Read the model definition and answer for the solid it produces. Units are mm, in the model's axes. Face numbers are marked on the shaded views. A direction names the side the tool comes from. Coordinates: 2 decimals unless noted, no trailing zeros. Loops run counter-clockwise (first coordinate to the right, second up) from the corner with the lowest first, then second, coordinate; pieces in that order, holes last. Notation, with made-up numbers: M -28,-35 L 22,-35 A26 ccw 22,-1 Z; hole C 19,52.25 d7. An arc over 180 degrees is marked long. Put each result on its own line as item: value.
from build123d import *

# Parameters (mm, degrees)
BOSS_EXTRUDE1_DEPTH = 46
BOSS_EXTRUDE2_DEPTH = 2
LPATTERN1_COUNT     = 6
LPATTERN1_PITCH     = 7.5
SKETCH3_W           = 10
SKETCH3_H           = 4
BOSS_EXTRUDE3_DEPTH = 8
CUT_EXTRUDE1_REACH  = 6
SKETCH4_R           = 1.55
FILLET1_R           = 3


with BuildPart() as part:
    # Sketch1 → Boss-Extrude1 (new body)
    with BuildSketch(Plane.XY):
        Polygon((0, 0), (0, 42), (-10, 42), (-20, 0), align=None)
    extrude(amount=BOSS_EXTRUDE1_DEPTH)

    # Sketch2 → Boss-Extrude2 (add)
    with BuildSketch(Plane.XY.offset(42.75)):
        with BuildLine():
            Line((-10.595238095, 39.5), (-20.5, 39.5))
            ThreePointArc((-20.5, 39.5), (-21.560660172, 39.060660172), (-22, 38))
            Line((-22, 38), (-22, 1.5))
            ThreePointArc((-22, 1.5), (-21.560660172, 0.439339828), (-20.5, 0))
            Line((-20.5, 0), (-20, 0))
            Line((-20, 0), (-10.595238095, 39.5))
        make_face()
    boss_extrude2 = extrude(amount=-BOSS_EXTRUDE2_DEPTH)

    # LPattern1: Boss-Extrude2 ×6
    with Locations(*[(0, 0, -i * LPATTERN1_PITCH) for i in range(1, LPATTERN1_COUNT)]):
        add(boss_extrude2)

    # Sketch3 → Boss-Extrude3 (add, symmetric)
    with BuildSketch(Plane.XY.offset(23)):
        with Locations((5, 2)):
            Rectangle(SKETCH3_W, SKETCH3_H)
    extrude(amount=BOSS_EXTRUDE3_DEPTH, both=True)

    # Sketch4 → Cut-Extrude1 (cut, up to next)
    with BuildSketch(Plane(origin=(0, 4, 0), x_dir=(1, 0, 0), z_dir=(0, 1, 0)), mode=Mode.PRIVATE) as cut_extrude1_sk1:
        with Locations((5, -19)):
            Circle(SKETCH4_R)
    cut_extrude1_tool1 = extrude(cut_extrude1_sk1.sketch, amount=-CUT_EXTRUDE1_REACH, mode=Mode.PRIVATE) & part.part
    add(cut_extrude1_tool1.solids().sort_by_distance((5, 4, 19))[0], mode=Mode.SUBTRACT)
    # Sketch4 → Cut-Extrude1 (cut, up to next)
    with BuildSketch(Plane(origin=(0, 4, 0), x_dir=(1, 0, 0), z_dir=(0, 1, 0)), mode=Mode.PRIVATE) as cut_extrude1_sk2:
        with Locations((5, -27)):
            Circle(SKETCH4_R)
    cut_extrude1_tool2 = extrude(cut_extrude1_sk2.sketch, amount=-CUT_EXTRUDE1_REACH, mode=Mode.PRIVATE) & part.part
    add(cut_extrude1_tool2.solids().sort_by_distance((5, 4, 27))[0], mode=Mode.SUBTRACT)

    # Fillet1
    fillet1_edges = [part.edges().sort_by_distance(p)[0] for p in [
        (10, 2, 15),
        (10, 2, 31),
    ]]
    fillet(fillet1_edges, radius=FILLET1_R)


solid = part.part
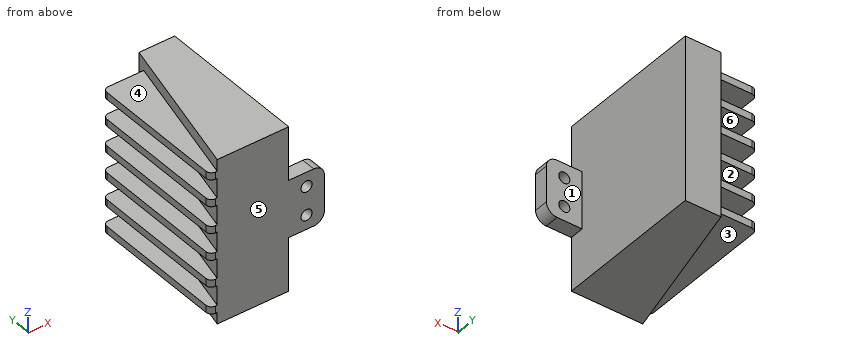
1) Find section D-D, the plane x = -15. Write down the section's boundary in (y, z), plus the area to 3 significant figures.
Answer list:
outline: M 0,0 L 21,0 L 21,3.25 L 39.5,3.25 L 39.5,5.25 L 21,5.25 L 21,10.75 L 39.5,10.75 L 39.5,12.75 L 21,12.75 L 21,18.25 L 39.5,18.25 L 39.5,20.25 L 21,20.25 L 21,25.75 L 39.5,25.75 L 39.5,27.75 L 21,27.75 L 21,33.25 L 39.5,33.25 L 39.5,35.25 L 21,35.25 L 21,40.75 L 39.5,40.75 L 39.5,42.75 L 21,42.75 L 21,46 L 0,46 Z
area: 1,190 mm^2
2) Which of the six approach directions +Z, -Z, +X, -X, +Y, -Y give full straight-line access (tool end or side, diameter ignored) to the marked faces 1, 2 and 3?
Answer list:
face 1: +Z, -Z, +X, +Y
face 2: -X, +Y
face 3: -Z, -X, +Y
3) Determine the mould class of the marked faces 4, 5 and 6 for opening direction Z: released by +Z, released by -Z, zero draft, split by the parting line, or undercut.
Answer list:
face 4: released by +Z
face 5: zero draft
face 6: undercut
4) Given pin 1 Ø10 at (y, z) = (10.5, 13.5) entering from -X; pin 2 Ø1 at (x, z) = (-17.5, 19.5) entering from +Y; pin 3 Ø3 at (x, y) = (4.5, 1.5) entering from +Z; pin 4 Ø5 at (x, z) = (4, 25.5) entering from +Y, each flat-ended and moving along its own axis, determine where each tip first touches the part or whether it passes through.
Answer list:
pin 1: stops at x = -22
pin 2: stops at y = 39.5
pin 3: stops at z = 31
pin 4: stops at y = 4
5) Find section B-B, the plane x = 5. Write down the section's boundary in (y, z), plus the area to 3 significant figures.
Answer list:
outline: M 0,15 L 4,15 L 4,17.45 L 0,17.45 Z; M 0,20.55 L 4,20.55 L 4,25.45 L 0,25.45 Z; M 0,28.55 L 4,28.55 L 4,31 L 0,31 Z
area: 39.2 mm^2
6) Find section C-C, the plane y = 25. Write down the section's boundary in (x, z).
Answer list:
outline: M -22,3.25 L -14.05,3.25 L -14.05,0 L 0,0 L 0,46 L -14.05,46 L -14.05,42.75 L -22,42.75 L -22,40.75 L -14.05,40.75 L -14.05,35.25 L -22,35.25 L -22,33.25 L -14.05,33.25 L -14.05,27.75 L -22,27.75 L -22,25.75 L -14.05,25.75 L -14.05,20.25 L -22,20.25 L -22,18.25 L -14.05,18.25 L -14.05,12.75 L -22,12.75 L -22,10.75 L -14.05,10.75 L -14.05,5.25 L -22,5.25 Z
7) Find section A-A, the plane z = 27. Write down the section's boundary in (x, y), plus the area to 3 significant figures.
Answer list:
outline: M -22,1.5 A1.5 ccw -20.5,0 L 3.45,0 L 3.45,4 L 0,4 L 0,42 L -10,42 L -10.6,39.5 L -20.5,39.5 A1.5 ccw -22,38 Z; M 6.55,0 L 10,0 L 10,4 L 6.55,4 Z
area: 921 mm^2
8) Straight lines are drawn through the part: line 1 (Z direction, x = 5, y = 1); line 2 (Z direction, x = -20, y = 8.5); line 3 (X direction, y = 1.35, z = 27). For each, find the intervals that lie inside material, in ascending order. Write a range as [from, to].
Answer list:
line 1: z = [15, 17.45], [20.55, 25.45], [28.55, 31]
line 2: z = [3.25, 5.25], [10.75, 12.75], [18.25, 20.25], [25.75, 27.75], [33.25, 35.25], [40.75, 42.75]
line 3: x = [-21.99, 3.45], [6.55, 10]
